Here's the drawing with two shaded views (mm, measured from the low corner). I have some questions. A direction names the side the tool comes from. Round coordinates to 2 decimals unless told otherwise and drop trailing zeros. Loops run counter-clockwise (first coordinate to the right, second up) from the corner with the lowest first, then second, coordinate; pieces in that order, holes last. Notation, with made-up numbers: (85, 16) -> (144, 16) arc R23 ccw to (144, 31) -> close; hole circle Ø6 at (-17, -16). An arc over 180 degrees is marked (long way). Use a Markdown table: item, result.
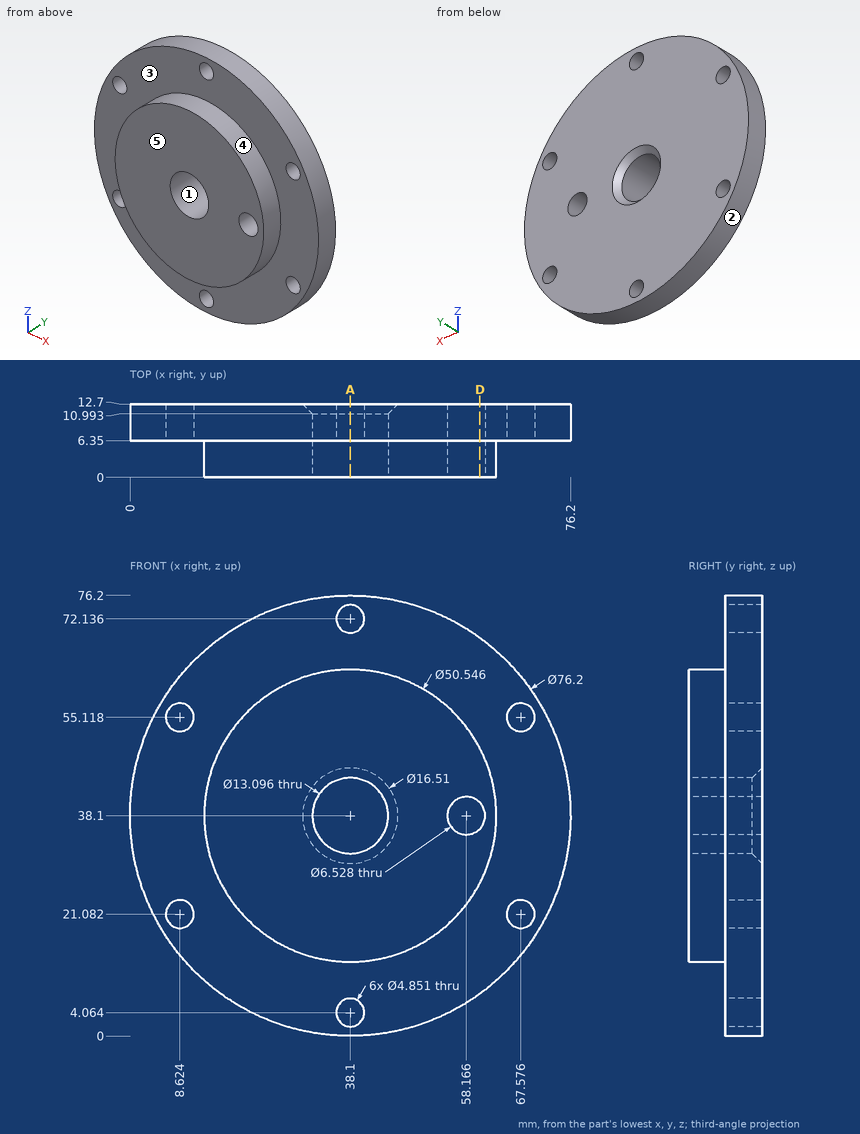
1. Will these pins go through, and if not, where does the flat tip stop? pin 1 Ø3 at (y, z) = (6.5, 54) entering from +X; pin 2 Ø4 at (y, z) = (6, 46) entering from +X (1 decimal); pin 3 Ø1.5 at (x, y) = (26.5, 3) entering from -Z (1 decimal).
Answer sheet:
| item | result |
|---|---|
| pin 1 | stops at x = 73.37 |
| pin 2 | stops at x = 75.7 |
| pin 3 | stops at z = 15.3 |
2. I want a section at D-D (x = 60.5). Please give me the cut outline in (y, z).
Answer sheet:
| item | result |
|---|---|
| outline | (0, 26.4) -> (6.35, 26.4) -> (6.35, 7.28) -> (12.7, 7.28) -> (12.7, 35.82) -> (0, 35.82) -> close; (0, 40.38) -> (12.7, 40.38) -> (12.7, 68.92) -> (6.35, 68.92) -> (6.35, 49.8) -> (0, 49.8) -> close |
3. I want a section at A-A (x = 38.1). State how many separate pieces and enclosed holes the cut face has, plus the area to 3 significant figures.
Answer sheet:
| item | result |
|---|---|
| separate pieces | 4 |
| enclosed holes | 0 |
| area | 574 mm² |
4. If we mould it in two halves opening along X, with no side actions, what happens to the marked faces 1, 2 and 3? For each: +X half, -X half, draft (parallel to the pull), parting line (faces both ways), or undercut.
Answer sheet:
| item | result |
|---|---|
| face 1 | undercut |
| face 2 | parting line |
| face 3 | draft |
5. Which directions (+Z, -Z, +X, -X, +Y, -Y) give clear straight access to the entire face, cutting with the end or side of a thin tool? Please do the marked faces 4 and 5.
Answer sheet:
| item | result |
|---|---|
| face 4 | -Y |
| face 5 | +Z, -Z, +X, -X, -Y |
6. I need wall thicknesses on line 1 (X direction, y = 8.25, z = 38.1); line 2 (X direction, y = 4.25, z = 38.1); line 3 (Z direction, x = 56, y = 9.5) (1 decimal). Which ranges of each line are inside material? Lowest first, please.
Answer sheet:
| item | result |
|---|---|
| line 1 | x = 0 to 31.55, 44.65 to 54.9, 61.43 to 76.2 |
| line 2 | x = 12.83 to 31.55, 44.65 to 54.9, 61.43 to 63.37 |
| line 3 | z = 4.5 to 35.7, 40.5 to 71.7 |
